Study the drawing (mm; zero at the part's minimum x, y, z) and answer. A direction names the side the tool comes from. Give positions to 0.01 mm unless a question says otherwise; leave off trailing zeros. Order: outer loops, then holes, each group sorted by start corner. A loop starts at its lowest first (then second) coordinate and runs counter-clockwise, first axis right, second up. Notation, with made-up numbers: (-6, -26) - (14, -26) arc R13 ccw to (14, -20) - close; hole circle Ø7 at (81, -7.75). An arc over 180 degrees is marked (long way). Write each question's results on one line, items separated by ' | '. Start each with the question number.
1. Section B-B (x = 8.25) is taken. Give the vertices of the cut face in (y, z).
2. Section C-C (z = 2.75) is taken. Give the vertices of the cut face in (x, y) (1 decimal).
3. Flat-ended cylindrical pins translate along their axes: pin 1 (0.9 mm diameter, centred on x = 16, z = 4, fed in from -Y); pin 2 (1 mm diameter, centred on x = 9.5, y = 13, fed in from +Z); pin 3 (0.9 mm diameter, centred on y = 3.5, z = 0.5, fed in from +X). Find the tip coordinate at first contact, or state that the pin passes through.
4. Find the intervals of material crossed by L1, parallel to X at y = 21, z = 3.25; L2, parallel to Z at x = 3.25, y = 9.5, in increasing order.
5. Section A-A (y = 25) is taken. Give the vertices of the cut face in (x, z).
6. Which of the six approach directions +Z, -Z, +X, -X, +Y, -Y give full straight-line access (tool end or side, diameter ignored) to the marked faces 1 and 2?
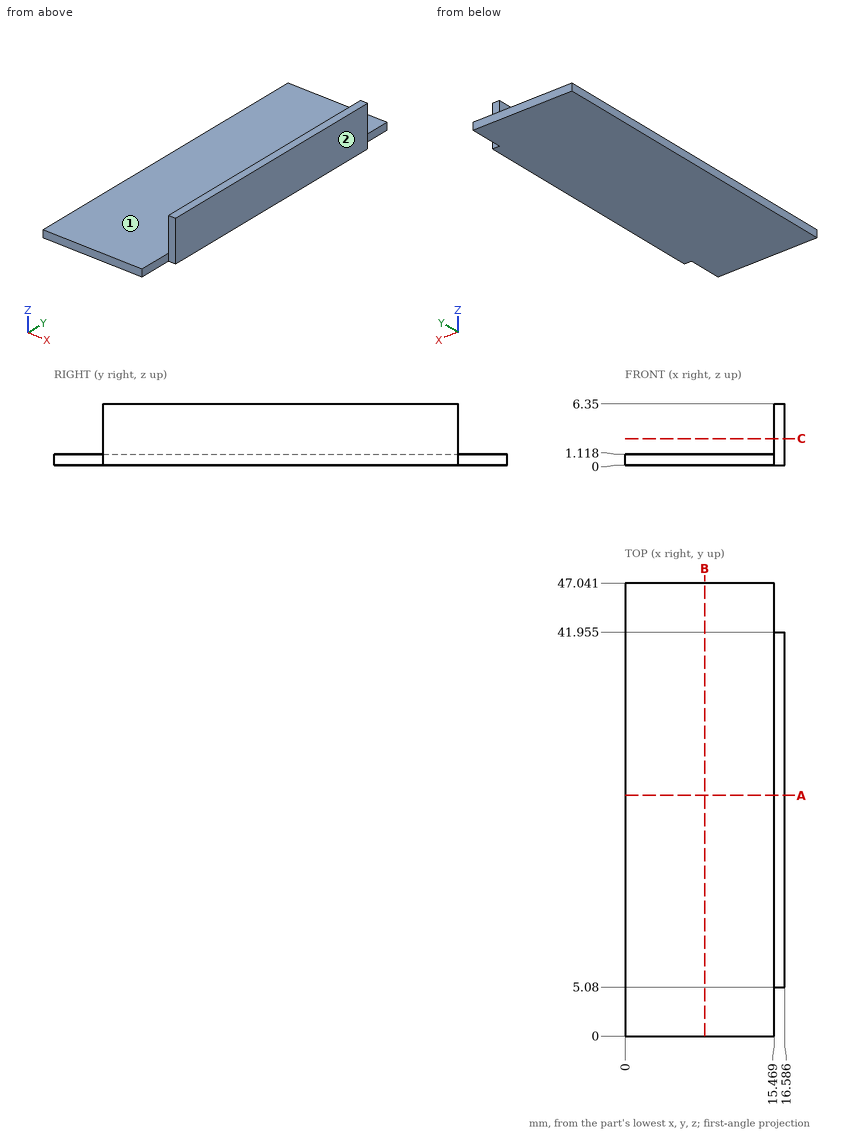
Reported:
1) outline: (0, 0) - (47.04, 0) - (47.04, 1.12) - (0, 1.12) - close
2) outline: (15.5, 5.1) - (16.6, 5.1) - (16.6, 42) - (15.5, 42) - close
3) pin 1: y = 5.08 | pin 2: z = 1.12 | pin 3: x = 15.47
4) L1: 15.47 to 16.59 | L2: 0 to 1.12
5) outline: (0, 0) - (16.59, 0) - (16.59, 6.35) - (15.47, 6.35) - (15.47, 1.12) - (0, 1.12) - close
6) face 1: +Z, -X, +Y, -Y | face 2: +Z, -Z, +X, +Y, -Y
